For this review, take the finished solid that the model builds, in its own axes (mm). Face numbers are marked on the shaded views. Round coordinates to 2 decimals unless told otherwise and drop trailing zeros. Write each loop counter-clockwise with the first axis right and the second up, starting at its lowest first coordinate (ties: lowest second). Pieces come first, ordered by that corner, then holes. Notation, with made-up numbers: (78, -7) -> (88, -7) arc R35 cw to (88, 29) -> close; hole circle Ø10 at (15.25, -12). An arc over 180 degrees is marked (long way). Write each question's results on one line, items separated by ' | '. Start each with the question number.
Item 1: Add section A-A (x = 0). State the section outline as (y, z) points, plus the area to 3 significant figures.
Item 2: Clearance check with flat-ended pins moving along their axes: pin 1 (1.5 mm diameter, centred on y = 8.5, z = -0.5, fed in from -X); pin 2 (1 mm diameter, centred on y = 5, z = 0, fed in from -X); pin 3 (3 mm diameter, centred on y = 12, z = 3.5, fed in from -X). State where each tip first meets the part, or that it passes through.
Item 3: To check wall thickness, follow line 1 along Z through (x, y) = (8.75, 2.25); line 2 along X through (y, z) = (7, 2.5); line 3 along Z through (x, y) = (0, 14). State the ranges of each line that lie inside material, in increasing order.
Item 4: Add section B-B (z = -5.5). State the section outline as (x, y) points.
Item 5: The part is to be moulded in two halves that separate along X. For the marked faces 1 and 2, say which applies: +X half, -X half, draft (parallel to the pull), parting line (faces both ways), or undercut.
Item 6: Add section C-C (z = 1). State the section outline as (x, y) points.
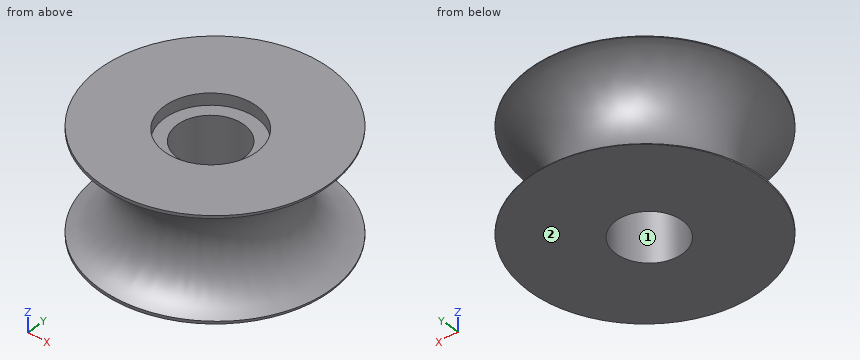
Autodesk Inventor part; units mm, degrees
ref_plane "YZ Plane" through (0, 0, 0) normal (1, 0, 0) x (0, 1, 0)
ref_plane "XZ Plane" through (0, 0, 0) normal (0, 1, 0) x (-1, 0, 0)
ref_plane "XY Plane" through (0, 0, 0) normal (0, 0, 1) x (1, 0, 0)
sketch "Sketch1" plane through (0, 0, 0) normal (1, 0, 0) x (0, 1, 0)
  line L0 (-6.098, -7.32) -> (9.142, -7.32)
  line L1 (9.142, 5.08) -> (-6.098, 5.08)
  line L2 (9.142, 6.8113) -> (9.142, -7.738)
  arc A0 (-6.098, -7.32) -> (-6.098, 5.08) centre (-6.098, -1.12) ccw
  point P0 (0, 0)
  dimension "d4" = 12.4
  dimension "d5" = 15.24
revolve "Revolution1" add sketch "Sketch1" angle 360 about axis through (0, 9.142, 6.8113) along (0, 0, -1)
sketch "Sketch2" plane through (0, 9.142, -7.32) normal (0, 0, -1) x (-1, 0, 0)
  circle A0 centre (0, 0) radius 15.24
  circle A1 centre (0, 0) radius 3.9688
  dimension "d1" = 7.9375
extrude "Extrusion1" cut sketch "Sketch2" against normal through all contours A1
sketch "Sketch4" plane through (0, 0, 0) normal (1, 0, 0) x (0, 1, 0)
  line L0 (23.5043, 7.0392) -> (26.3008, 7.0392)
  line L1 (26.3008, 7.0392) -> (26.3008, -7.7625)
  line L2 (26.3008, -7.7625) -> (23.5043, -7.7625)
  line L3 (23.5043, -7.7625) -> (23.5043, 7.0392)
  line L4 (9.7561, -8.4) -> (9.7561, 8.96)
  point P0 (0, 0)
revolve "Revolution2" cut sketch "Sketch4" angle 360 about axis through (0, 9.7561, -8.4) along (0, 0, 1)
sketch "Sketch5" plane through (0, 9.7561, 5.08) normal (0, 0, 1) x (1, 0, 0)
  circle A0 centre (0, -0.6141) radius 5.5
  point P0 (0, -9.7561)
extrude "Extrusion3" cut sketch "Sketch5" against normal blind 1.4
properties part number "surgicalpulley"
Responses:
1) outline: (-3.99, -7.32) -> (5.17, -7.32) -> (5.17, 3.68) -> (3.64, 3.68) -> (3.64, 5.08) -> (-3.99, 5.08) -> (-3.99, 4.71) arc R6.2 cw to (-3.99, -6.95) -> close; (13.11, -7.32) -> (23.5, -7.32) -> (23.5, -7.26) arc R6.2 cw to (23.5, 5.02) -> (23.5, 5.08) -> (14.64, 5.08) -> (14.64, 3.68) -> (13.11, 3.68) -> close | area: 154 mm^2
2) pin 1: stops at x = -9.18 | pin 2: stops at x = -8.41 | pin 3: stops at x = -13.64
3) line 1: z = -7.32 to -5.77, 3.53 to 5.08 | line 2: x = -9.98 to -3.34, 3.34 to 9.98 | line 3: z = -7.32 to 3.68
4) outline: circle Ø21.7 at (0, 9.14); hole circle Ø7.94 at (0, 9.14)
5) face 1: undercut | face 2: draft
6) outline: circle Ø18.83 at (0, 9.14); hole circle Ø7.94 at (0, 9.14)
